from build123d import *

# Parameters (mm, degrees)
F0_W     = 98.028793931
F0_H     = 57.4665814638
F1_DEPTH = 25.4
F2_SIZE  = 25.39999
F3_SIZE  = 25.39999
F4_DEPTH = 86.0725715756


# Not quite as in the source:
# - a fillet or chamfer is up to 0.001 mm smaller than in the source, because OpenCascade refuses the exact size


with BuildPart() as f1:
    # F0 (on Top) → F1 (new body)
    with BuildSketch(Plane.XY):
        with Locations((1.7422363162, 28.7332907319)):
            Rectangle(F0_W, F0_H)
    extrude(amount=F1_DEPTH)

    # F2 (size 25.4 in the source; OpenCascade refuses exactly that, so slightly less here)
    f2_edges = [f1.edges().sort_by_distance(p)[0] for p in [
        (50.756633, 28.733291, 25.4),
    ]]
    chamfer(f2_edges, length=F2_SIZE)

    # F3 (size 25.4 in the source; OpenCascade refuses exactly that, so slightly less here)
    f3_edges = [f1.edges().sort_by_distance(p)[0] for p in [
        (-47.272161, 28.733291, 25.4),
    ]]
    chamfer(f3_edges, length=F3_SIZE)

    # F4 (add): a face of the model
    f4_faces = [f1.faces().sort_by_distance(p)[0] for p in [
        (1.7422363162, 28.7332907319, 0),
    ]]
    extrude(f4_faces, amount=F4_DEPTH)


solid = f1.part
Work out the finished part from the listing and answer in its coordinate system (mm). Give positions to 0.01 mm unless a question says otherwise; leave off trailing zeros. Write each loop counter-clockwise with the first axis right and the second up, starting at its lowest first coordinate (ties: lowest second). Pieces come first, ordered by that corner, then holes. Notation, with made-up numbers: (13.25, 67) - (37.25, 67) arc R18 ccw to (37.25, 102) - close; hole circle Ø6 at (-3.75, 26.5). An arc over 180 degrees is marked (long way). One line per item, written item: value. Start each with the question number.
1. Find section A-A (y = 7). Write down the section's boundary in (x, z), then the cut area to 3 significant figures.
2. Consider probe 1 along Z at (x, y) = (37.5, 25.5); probe 2 along Z at (x, y) = (27.5, 11); probe 3 along X at (y, z) = (22.5, 9.5). Determine where each line is inside the solid, lowest interval first.
3. Find section C-C (z = 18.5). Write down the section's boundary in (x, y).
4. Given pin 1 (12 mm diameter, centred on x = 32, y = 16.5, fed in from +Z); pin 2 (1.5 mm diameter, centred on x = -37, y = 10.5, fed in from +Z), each flat-ended and moving along its own axis, determine where each tip first touches the part or whether it passes through.
5. Find section B-B (x = 38.5). Write down the section's boundary in (y, z), then the cut area to 3 significant figures.
Geometry results:
1. outline: (-47.27, -86.07) - (50.76, -86.07) - (50.76, 0) - (25.36, 25.4) - (-21.87, 25.4) - (-47.27, 0) - close
1. area: 10,300 mm2
2. probe 1: -86.07 to 13.26
2. probe 2: -86.07 to 23.26
2. probe 3: -37.77 to 41.26
3. outline: (-28.77, 0) - (32.26, 0) - (32.26, 57.47) - (-28.77, 57.47) - close
4. pin 1: z = 24.76
4. pin 2: z = 11.02
5. outline: (0, -86.07) - (57.47, -86.07) - (57.47, 12.26) - (0, 12.26) - close
5. area: 5,650 mm2
